from build123d import *

# Parameters (mm, degrees)
CROQUIS1_R              = 1.2
SALIENTE_EXTRUIR1_DEPTH = 5.95
CROQUIS2_R              = 1.425
SALIENTE_EXTRUIR2_DEPTH = 3


with BuildPart() as part:
    # Croquis1 → Saliente-Extruir1 (new body)
    with BuildSketch(Plane.XY):
        Polygon((0, -2.684678752), (2.325, -1.342339376), (2.325, 1.342339376), (0, 2.684678752), (-2.325, 1.342339376), (-2.325, -1.342339376), align=None)
        Circle(CROQUIS1_R, mode=Mode.SUBTRACT)
    extrude(amount=SALIENTE_EXTRUIR1_DEPTH)

    # Croquis2 → Saliente-Extruir2 (add)
    with BuildSketch(Plane.XY.offset(5.95)):
        Circle(CROQUIS2_R)
    extrude(amount=SALIENTE_EXTRUIR2_DEPTH)


solid = part.part
Verification items for the finished model (mm, model axes). A direction names the side the tool comes from. Coordinates: 2 decimals unless noted, no trailing zeros. Order: outer loops, then holes, each group sorted by start corner. A loop starts at its lowest first (then second) coordinate and runs counter-clockwise, first axis right, second up. Notation, with made-up numbers: (71, 61.5) -> (112, 61.5) arc R22 ccw to (112, 71.5) -> close; hole circle Ø1 at (-39.75, -5.5). An arc over 180 degrees is marked (long way). Put each result on its own line as item: value. Start each with the question number.
1. Go/stop test with flat-tipped pins: pin 1 Ø1 at (y, z) = (0.5, 8) entering from -X (3 decimals); pin 2 Ø2 at (x, z) = (0.5, 3.5) entering from -Y; pin 3 Ø1.4 at (x, y) = (0, 0) entering from -Z. Record where each tip stops, or that it passes through.
2. Access from +Z, -Z, +X, -X, +Y, -Y to the whole of each face (thin tool, end or side, straight path). Record for faces 4 (the cylindrical face through (0.65, 1.01, 2.93)), 5 (the cylindrical face through (-1.13, -0.87, 7.43)), 6 (the flat face through (-1.15, 2.02, 2.93)).
3. Cross-section at C-C, the plane z = 6.25. Record the boundary of the cut face in (x, y) (3 decimals), then the cut area to 3 significant figures.
4. Cross-section at A-A, the plane z = 3. Record the boundary of the cut face in (x, y) (3 decimals).
5. Cross-section at B-B, the plane y = 0. Record the boundary of the cut face in (x, z) (3 decimals).
6. Material ranges on L1, parallel to Z at x = -2.1, y = 1.2; L2, parallel to Y at x = -0.05, z = 4.5; L3, parallel to Y at x = -1, z = 2.5, recorded low to high. Write a range as [from, to].
7. Mould release check, pull along Y, two halves, no side actions. Record for faces 1 (the flat face through (2.325, 0, 3)), 2 (the flat face through (0, 0, 5.95)), 3 (the flat face through (-1.179, -2.004, 2.933)): released by +Y, released by -Y, zero draft, split by the parting line, or undercut.
8. Cross-section at D-D, the plane x = -1.65. Record the boundary of the cut face in (y, z), then the cut area to 3 significant figures.
Computed:
1. pin 1: x = -1.425
1. pin 2: y = -2.68
1. pin 3: z = 5.95
2. face 4: -Z
2. face 5: +Z
2. face 6: +Z, -Z, -X, +Y
3. outline: circle Ø2.85 at (0, 0)
3. area: 6.38 mm2
4. outline: (-2.325, -1.342) -> (0, -2.685) -> (2.325, -1.342) -> (2.325, 1.342) -> (0, 2.685) -> (-2.325, 1.342) -> close; hole circle Ø2.4 at (0, 0)
5. outline: (-2.325, 0) -> (-1.2, 0) -> (-1.2, 5.95) -> (1.2, 5.95) -> (1.2, 0) -> (2.325, 0) -> (2.325, 5.95) -> (1.425, 5.95) -> (1.425, 8.95) -> (-1.425, 8.95) -> (-1.425, 5.95) -> (-2.325, 5.95) -> close
6. L1: [0, 5.95]
6. L2: [-2.66, -1.2], [1.2, 2.66]
6. L3: [-2.11, -0.66], [0.66, 2.11]
7. face 1: zero draft
7. face 2: undercut
7. face 3: released by -Y
8. outline: (-1.73, 0) -> (1.73, 0) -> (1.73, 5.95) -> (-1.73, 5.95) -> close
8. area: 20.6 mm2
